```python
from build123d import *

# Parameters (mm, degrees)
BOSS_EXTRUDE1_DEPTH = 10


with BuildPart() as part:
    # Sketch1 → Boss-Extrude1 (new body)
    with BuildSketch(Plane(origin=(0, 0, 0), x_dir=(0, 0, -1), z_dir=(1, 0, 0))):
        with BuildLine():
            Line((10, -5), (3.31662479, -5))
            ThreePointArc((3.31662479, -5), (0, 6), (-3.31662479, -5))
            Line((-3.31662479, -5), (-10, -5))
            Line((-10, -5), (-10, -6))
            Line((-10, -6), (-0.597061761, -6))
            Line((-0.597061761, -6), (-0.597061761, -4.964223731))
            ThreePointArc((-0.597061761, -4.964223731), (0.062391283, 4.999610718), (0.472995759, -4.977577223))
            Line((0.472995759, -4.977577223), (0.472995759, -6))
            Line((0.472995759, -6), (10, -6))
            Line((10, -6), (10, -5))
        make_face()
    extrude(amount=BOSS_EXTRUDE1_DEPTH)


solid = part.part
```
Could you check a few things on this model? Use its own coordinates, in mm. A direction names the side the tool comes from. Give positions to 0.01 mm unless a question says otherwise; leave off trailing zeros. Loops run counter-clockwise (first coordinate to the right, second up) from the corner with the lowest first, then second, coordinate; pieces in that order, holes last. Notation, with made-up numbers: (69, 73.5) - (117, 73.5) arc R27 cw to (117, 112.5) - close; hole circle Ø1 at (86.5, -33.5). An arc over 180 degrees is marked (long way). Answer in a Markdown table with one row per item. Add a question column.
Q1. If we section it at B-B (x = 6.75): List the corners of the cut face in (y, z) for me.
Q2. For pin 1 (4 mm diameter, centred on x = 2.5, y = 0.5, fed in from +Z); pin 2 (5.5 mm diameter, centred on x = 2.5, z = 8, fed in from +Y), each with a flat end and sliding along its axis, tell me the tip position at first contact or that it passes through.
Q3. We'd pull the mould along Y, two halves only. Please class faces 4 (the face through (5, -6, -5)), 5 (the face through (4.9, -5.5, 10)), 6 (the face through (5, -5, -7)), 7 (the face through (5, 5, 0)): +Y half, -Y half, draft (parallel to the pull), parting line (faces both ways), or undercut.
Q4. If we section it at D-D (z = -6.75): List the corners of the cut face in (x, y) for me.
Q5. If we section it at A-A (y = 0): List the corners of the cut face in (x, z) for me, plus the area to 3 significant figures.
Q6. If we section it at C-C (z = -3): List the corners of the cut face in (x, y) for me.
Q7. Please list where these lines run through material, in increasing order: L1, parallel to Z at x = 4, y = 0; L2, parallel to Z at x = 8.5, y = -5.25; L3, parallel to Y at x = 8, z = 0. Write a range as from..to.
Q8. Which directions (+Z, -Z, +X, -X, +Y, -Y) give clear straight access to the entire face, cutting with the end or side of a thin tool? Please do faces 1 (the face through (4.9, -5.5, -0.473)), 2 (the face through (0, -5.3, -0.7)), 3 (the face through (5, -5, 7)).
The answers:
| question | item | result |
|---|---|---|
| 1 | outline | (-6, -10) - (-5, -10) - (-5, -3.32) arc R6 ccw (long way) to (-5, 3.32) - (-5, 10) - (-6, 10) - (-6, 0.6) - (-4.96, 0.6) arc R5 cw (long way) to (-4.98, -0.47) - (-6, -0.47) - close |
| 2 | pin 1 | stops at z = 6 |
| 2 | pin 2 | stops at y = 2.9 |
| 3 | face 4 | -Y half |
| 3 | face 5 | draft |
| 3 | face 6 | undercut |
| 3 | face 7 | undercut |
| 4 | outline | (0, -6) - (10, -6) - (10, -5) - (0, -5) - close |
| 5 | outline | (0, -6) - (10, -6) - (10, -5) - (0, -5) - close; (0, 5) - (10, 5) - (10, 6) - (0, 6) - close |
| 5 | area | 20.0 mm^2 |
| 6 | outline | (0, -6) - (10, -6) - (10, -4) - (0, -4) - close; (0, 4) - (10, 4) - (10, 5.2) - (0, 5.2) - close |
| 7 | L1 | z = -6..-5, 5..6 |
| 7 | L2 | z = -10..-0.47, 0.6..10 |
| 7 | L3 | y = 5..6 |
| 8 | face 1 | +X, -X, -Y |
| 8 | face 2 | +Z, -Z, -X, +Y, -Y |
| 8 | face 3 | +Z, +X, -X |
